Source: CAD feature listing. Evaluate the final solid. Frame: model axes, mm. A direction names the side the tool comes from. Round coordinates to 2 decimals unless told otherwise and drop trailing zeros. Loops run counter-clockwise (first coordinate to the right, second up) from the corner with the lowest first, then second, coordinate; pieces in that order, holes last. Notation, with made-up numbers: (74, 14) - (132, 14) arc R21 cw to (132, 48) - close; hole circle Ø9 at (-39.75, 17). An arc over 180 degrees is marked (long way). One line per question, with ' | ' between items. Start each with the question number.
1. Ray query, line 1 (Y direction, x = -7, z = -3); line 2 (Y direction, x = -4.5, z = 7.5); line 3 (X direction, y = -8, z = 15). Return the intervals inside material, ascending.
2. Cut plane C-C (z = -3). Return loops of the section in (x, y), then the cut area to 3 significant figures.
3. Mould query, pull axis Y, two halves, no side actions, for faces 1 (the flat face through (-4, -19.05, -4)), 2 (the flat face through (16, 10, -19.05)), 3 (the flat face through (12.7, 9, -10)). Classes: pulls with the +Y half, pulls with the -Y half, needs draft (parallel to the pull), parting line crosses it, or undercut.
4. Cut plane B-B (x = -1). Return loops of the section in (y, z).
5. Pin query (flat end, axial travel): pin 1 (5.5 mm diameter, centred on y = 9, z = -13.5, fed in from -X); pin 2 (15 mm diameter, centred on y = 27, z = 12.5, fed in from +X); pin 3 (21 mm diameter, centred on y = 32.5, z = 8, fed in from -X). Return the tip coordinate at first contact, or that it passes through.
6. Cut plane D-D (y = -9). Return loops of the section in (x, z), then the cut area to 3 significant figures.
7. Cut plane A-A (z = 12). Return loops of the section in (x, y).
8. Access query for faces 4 (the flat face through (12.7, 28, 9)), 5 (the flat face through (3, 19.05, 0)), 6 (the flat face through (-6.35, 28, 0)), 7 (the flat face through (-6.35, -9, 9)). Directions: +Z, -Z, +X, -X, +Y, -Y. A direction counts if a zero-diameter tool reaches every point of the face in a straight line with its end or side. Return the directions, or none.
```python
from build123d import *

# Parameters (mm, degrees)
F1_DEPTH = 19.05
F2_W     = 19.05
F2_H     = 19.05
F3_DEPTH = 38.1
F4_W     = 19.05
F4_H     = 19.05
F5_DEPTH = 19.05
F6_W     = 19.05
F6_H     = 19.05
F7_DEPTH = 19.05


with BuildPart() as f1:
    # F0 (on Front) → F1 (new body)
    with BuildSketch(Plane.XZ):
        Polygon((-25.4, 19.05), (-25.4, -19.05), (31.75, -19.05), (31.75, 0), (-6.35, 0), (-6.35, 19.05), align=None)
    extrude(amount=F1_DEPTH)

    # F2 (on face) → F3 (join)
    with BuildSketch(Plane(origin=(0, 0, 0), x_dir=(-1, 0, 0), z_dir=(0, 1, 0))):
        with Locations((-22.225, -9.525)):
            Rectangle(F2_W, F2_H)
    extrude(amount=F3_DEPTH)

    # F4 (on face) → F5 (join)
    with BuildSketch(Plane(origin=(12.7, 0, 0), x_dir=(0, -1, 0), z_dir=(-1, 0, 0))):
        with Locations((-28.575, -9.525)):
            Rectangle(F4_W, F4_H)
    extrude(amount=F5_DEPTH)

    # F6 (on face) → F7 (join)
    with BuildSketch(Plane.XY):
        with Locations((3.175, 28.575)):
            Rectangle(F6_W, F6_H)
    extrude(amount=F7_DEPTH)


solid = f1.part
```
Answers follow:
1) line 1: y = -19.05 to 0 | line 2: y = 19.05 to 38.1 | line 3: x = -25.4 to -6.35
2) outline: (-25.4, -19.05) - (31.75, -19.05) - (31.75, 38.1) - (-6.35, 38.1) - (-6.35, 19.05) - (12.7, 19.05) - (12.7, 0) - (-25.4, 0) - close | area: 2,180 mm2
3) face 1: pulls with the -Y half | face 2: needs draft | face 3: undercut
4) outline: (-19.05, -19.05) - (0, -19.05) - (0, 0) - (-19.05, 0) - close; (19.05, -19.05) - (38.1, -19.05) - (38.1, 19.05) - (19.05, 19.05) - close
5) pin 1: stops at x = 12.7 | pin 2: stops at x = 12.7 | pin 3: stops at x = -6.35
6) outline: (-25.4, -19.05) - (31.75, -19.05) - (31.75, 0) - (-6.35, 0) - (-6.35, 19.05) - (-25.4, 19.05) - close | area: 1,450 mm2
7) outline: (-25.4, -19.05) - (-6.35, -19.05) - (-6.35, 0) - (-25.4, 0) - close; (-6.35, 19.05) - (12.7, 19.05) - (12.7, 38.1) - (-6.35, 38.1) - close
8) face 4: +Z, +X, +Y, -Y | face 5: +Z, -Z, -X | face 6: +Z, -Z, -X, +Y | face 7: +Z, +X, -Y
